```python
from build123d import *

# Parameters (mm, degrees)
SKETCH1_R           = 54.61
SKETCH1_R_2         = 52.07
BOSS_EXTRUDE1_DEPTH = 25.4
SKETCH3_R           = 1.905
CUT_EXTRUDE1_DEPTH  = 55.61
CIRPATTERN1_COUNT   = 3


with BuildPart() as part:
    # Sketch1 → Boss-Extrude1 (new body)
    with BuildSketch(Plane(origin=(0, 0, 0), x_dir=(1, 0, 0), z_dir=(0, 1, 0))):
        Circle(SKETCH1_R)
        Circle(SKETCH1_R_2, mode=Mode.SUBTRACT)
    extrude(amount=BOSS_EXTRUDE1_DEPTH)

    # Sketch3 → Cut-Extrude1 (cut, through all)
    with BuildSketch(Plane.XY):
        with Locations((0, 12.328955527)):
            Circle(SKETCH3_R)
    cut_extrude1 = extrude(amount=CUT_EXTRUDE1_DEPTH, mode=Mode.SUBTRACT)

    # CirPattern1: Cut-Extrude1 ×3 about axis
    cirpattern1_axis = Axis((0, 25.4, 0), (0, 1, 0))
    for i in range(1, CIRPATTERN1_COUNT):
        add(cut_extrude1.rotate(cirpattern1_axis, i * 360 / CIRPATTERN1_COUNT), mode=Mode.SUBTRACT)


solid = part.part
```
CAD build for the part. Positions are in the model's coordinates, mm. A direction names the side the tool comes from. Coordinates: 2 decimals unless noted, no trailing zeros. Order: outer loops, then holes, each group sorted by start corner. A loop starts at its lowest first (then second) coordinate and runs counter-clockwise, first axis right, second up.
(1) Mould opens along Z. For faces 3 (the face through (46.37, 10.47, -26.29)), 4 (the face through (48.3, 25.4, 20)), 5 (the face through (-7.109, 12.522, -54.145)) say: released by +Z, released by -Z, zero draft, split by the parting line, or undercut.
Solution:
face 3: undercut
face 4: zero draft
face 5: split by the parting line
(2) Saw through at A-A, the plane z = 0. Write the cut outline in (x, y), and give its area (3 significant figures).
Solution:
outline: (-54.61, 0) - (-52.07, 0) - (-52.07, 25.4) - (-54.61, 25.4) - close; (52.07, 0) - (54.61, 0) - (54.61, 25.4) - (52.07, 25.4) - close
area: 129 mm2
(3) Drill centre lines: L1, parallel to Y at x = 0, z = 53.4; L2, parallel to Z at x = 0, y = 16.75. Where is each one in solid material? Low to high.
Solution:
L1: y = 0 to 10.42, 14.23 to 25.4
L2: z = -54.61 to -52.07, 52.07 to 54.61
(4) Which spindle directions (+Z, -Z, +X, -X, +Y, -Y) get a long thin tool onto all of the face, cutting with end or side? Do faces 1 (the face through (48.3, 0, 20)), 2 (the face through (-0.41, 10.47, 53.3)). Say none if no direction does.
Solution:
face 1: +Z, -Z, +X, -X, -Y
face 2: +Z
(5) Saw through at D-D, the plane y = 4. Write the cut outline in (x, z).
Solution:
outline: circle Ø109.22 at (0, 0); hole circle Ø104.14 at (0, 0)
(6) Saw through at C-C, the plane x = -12. Write the cut outline in (y, z), and give its area (3 significant figures).
Solution:
outline: (0, -53.28) - (25.4, -53.28) - (25.4, -50.67) - (0, -50.67) - close; (0, 50.67) - (25.4, 50.67) - (25.4, 53.28) - (0, 53.28) - close
area: 132 mm2
(7) Saw through at B-B, the plane x = 0. Write the cut outline in (y, z).
Solution:
outline: (0, -54.61) - (25.4, -54.61) - (25.4, -52.07) - (0, -52.07) - close; (0, 52.07) - (10.42, 52.07) - (10.42, 54.61) - (0, 54.61) - close; (14.23, 52.07) - (25.4, 52.07) - (25.4, 54.61) - (14.23, 54.61) - close
(8) Pin check, flat tips, straight feed: pin 1 Ø2 at (y, z) = (8.5, 42) entering from -X; pin 2 Ø1 at (y, z) = (7, 13.5) entering from -X; pin 3 Ø12 at (x, y) = (-9.5, 15.5) entering from -Z. Stop position of each tip, or through.
Solution:
pin 1: stops at x = -36.07
pin 2: stops at x = -53.04
pin 3: stops at z = -54.5
